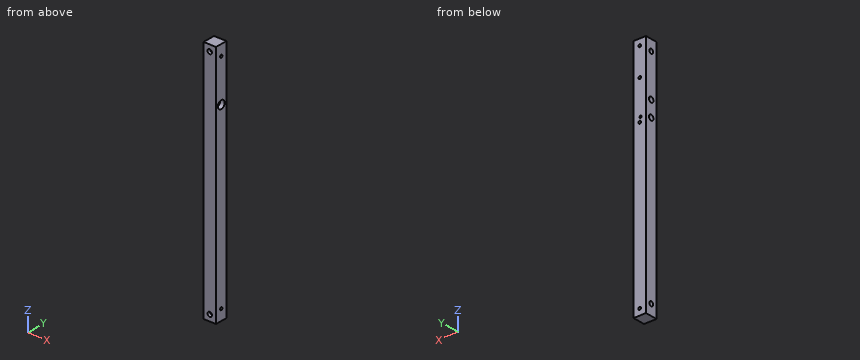
from build123d import *

# Parameters (mm, degrees)
IZIM1_W                     = 28
IZIM1_H                     = 28
Y_KSEKLIK_EKSTR_ZYON1_DEPTH = 270
IZIM3_R                     = 3
KES_EKSTR_ZYON2_DEPTH       = 272.808756298
IZIM4_R                     = 5
KES_EKSTR_ZYON3_DEPTH       = 7
IZIM5_R                     = 6
KES_EKSTR_ZYON4_DEPTH       = 272.808756298
IZIM6_R                     = 9
KES_EKSTR_ZYON5_DEPTH       = 10
IZIM7_R                     = 3
KES_EKSTR_ZYON6_DEPTH       = 272.808756298
IZIM8_R                     = 5
KES_EKSTR_ZYON7_DEPTH       = 7
SKETCH1_R                   = 3
CUT_EXTRUDE1_DEPTH          = 10
SKETCH2_R                   = 6
CUT_EXTRUDE2_DEPTH          = 20
SKETCH3_R                   = 2.5
CUT_EXTRUDE3_DEPTH          = 14


with BuildPart() as part:
    # Çizim1 → Yükseklik-Ekstrüzyon1 (new, symmetric)
    with BuildSketch(Plane.XY):
        Rectangle(IZIM1_W, IZIM1_H)
    extrude(amount=Y_KSEKLIK_EKSTR_ZYON1_DEPTH, both=True)

    # Çizim3 → Kes-Ekstrüzyon2 (cut, through all)
    with BuildSketch(Plane.XZ.offset(14)):
        with Locations(Location((0, -256, 0), (0, 0, 270))):
            Circle(IZIM3_R)
        with Locations(Location((0, 256, 0), (0, 0, 270))):
            Circle(IZIM3_R)
    extrude(amount=-KES_EKSTR_ZYON2_DEPTH, mode=Mode.SUBTRACT)

    # Çizim4 → Kes-Ekstrüzyon3 (cut)
    with BuildSketch(Plane.XZ.offset(14)):
        with Locations(Location((0, -256, 0), (0, 0, 270))):
            Circle(IZIM4_R)
        with Locations(Location((0, 256, 0), (0, 0, 270))):
            Circle(IZIM4_R)
    extrude(amount=-KES_EKSTR_ZYON3_DEPTH, mode=Mode.SUBTRACT)

    # Çizim5 → Kes-Ekstrüzyon4 (cut, through all)
    with BuildSketch(Plane(origin=(14, 0, 0), x_dir=(0, 0, -1), z_dir=(1, 0, 0))):
        with Locations((-151.8, 0)):
            Circle(IZIM5_R)
    extrude(amount=-KES_EKSTR_ZYON4_DEPTH, mode=Mode.SUBTRACT)

    # Çizim6 → Kes-Ekstrüzyon5 (cut)
    with BuildSketch(Plane(origin=(14, 0, 0), x_dir=(0, 0, -1), z_dir=(1, 0, 0))):
        with Locations((-151.8, 0)):
            Circle(IZIM6_R)
    extrude(amount=-KES_EKSTR_ZYON5_DEPTH, mode=Mode.SUBTRACT)

    # Çizim7 → Kes-Ekstrüzyon6 (cut, through all)
    with BuildSketch(Plane.ZY.offset(14)):
        with Locations((-246, 0)):
            Circle(IZIM7_R)
        with Locations((246, 0)):
            Circle(IZIM7_R)
    extrude(amount=-KES_EKSTR_ZYON6_DEPTH, mode=Mode.SUBTRACT)

    # Çizim8 → Kes-Ekstrüzyon7 (cut)
    with BuildSketch(Plane.ZY.offset(14)):
        with Locations((-246, 0)):
            Circle(IZIM8_R)
        with Locations((246, 0)):
            Circle(IZIM8_R)
    extrude(amount=-KES_EKSTR_ZYON7_DEPTH, mode=Mode.SUBTRACT)

    # Sketch1 → Cut-Extrude1 (cut)
    with BuildSketch(Plane(origin=(0, 14, 0), x_dir=(1, 0, 0), z_dir=(0, 1, 0))):
        with Locations(Location((0, -106.8, 0), (0, 0, 270))):
            Circle(SKETCH1_R)
        with Locations(Location((0, -193.8, 0), (0, 0, 270))):
            Circle(SKETCH1_R)
    extrude(amount=-CUT_EXTRUDE1_DEPTH, mode=Mode.SUBTRACT)

    # Sketch2 → Cut-Extrude2 (cut)
    with BuildSketch(Plane.ZY.offset(14)):
        with Locations((116.8, 0)):
            Circle(SKETCH2_R)
    extrude(amount=-CUT_EXTRUDE2_DEPTH, mode=Mode.SUBTRACT)

    # Sketch3 → Cut-Extrude3 (cut)
    with BuildSketch(Plane(origin=(0, 14, 0), x_dir=(1, 0, 0), z_dir=(0, 1, 0))):
        with Locations(Location((-2, -116.8, 0), (0, 0, 270))):
            Circle(SKETCH3_R)
    extrude(amount=-CUT_EXTRUDE3_DEPTH, mode=Mode.SUBTRACT)


solid = part.part
For this review, take the finished solid that the model builds, in its own axes (mm). Round coordinates to 2 decimals unless told otherwise and drop trailing zeros. Order: outer loops, then holes, each group sorted by start corner. A loop starts at its lowest first (then second) coordinate and runs counter-clockwise, first axis right, second up. Notation, with made-up numbers: (14, 76.25) -> (35, 76.25) arc R7 ccw to (35, 86.25) -> close; hole circle Ø8 at (82, -6.5). An arc over 180 degrees is marked (long way). Put each result on its own line as item: value.
Q1. Add section A-A on z = 151.8. Write out the cut boundary in (x, y).
Check result:
outline: (-14, -14) -> (14, -14) -> (14, -9) -> (4, -9) -> (4, -6) -> (-14, -6) -> close; (-14, 6) -> (4, 6) -> (4, 9) -> (14, 9) -> (14, 14) -> (-14, 14) -> close
Q2. Insertion check: pin 1 Ø5.5 at (x, z) = (0, 193.8) entering from +Y; pin 2 Ø5.5 at (y, z) = (0, 246) entering from +X; pin 3 Ø9.5 at (y, z) = (0.5, 117.5) entering from -X; pin 4 Ø9 at (x, z) = (0, 256) entering from -Y. Each pin has a flat end and moves straight along its axis. Give the tip position at first contact, or say it passes through.
Check result:
pin 1: y = 4
pin 2: through
pin 3: x = 6
pin 4: y = -7
Q3. For probe 1 along Y at (x, z) = (-5.5, 116.8); probe 2 along Z at (x, y) = (-10.5, 2); probe 3 along Y at (x, z) = (-9, 246), list the stretches that pass through material, from the lowest coordinate up. Write a range as [from, to].
Check result:
probe 1: [-14, -6], [6, 14]
probe 2: [-270, -250.58], [-241.42, 111.14], [122.46, 146.14], [157.46, 241.42], [250.58, 270]
probe 3: [-14, -5], [5, 14]
